from build123d import *

# Parameters (mm, degrees)
SKETCH_1_R      = 2.8
EXTRUDE_1_DEPTH = 8
SKETCH_2_W      = 18.05
SKETCH_2_H      = 18.05
EXTRUDE_2_DEPTH = 1
SKETCH_3_W      = 18.05
SKETCH_3_H      = 18.05
SKETCH_3_W_2    = 16.05
SKETCH_3_H_2    = 16.05
EXTRUDE_3_DEPTH = 9
SKETCH_6_W      = 1.2
SKETCH_6_H      = 5.825
SKETCH_6_W_2    = 5.825
SKETCH_6_H_2    = 1.2
EXTRUDE_4_DEPTH = 2.5
FILLET_3_R      = 5
FILLET_4_R      = 1.6


with BuildPart() as part:
    # 草图1 → 凸台-拉伸1 (new body)
    with BuildSketch(Plane(origin=(0, 0, 0), x_dir=(1, 0, 0), z_dir=(0, 1, 0))):
        with Locations(Location((0, 0, 0), (0, 0, 270))):
            Circle(SKETCH_1_R)
        Polygon((2.2, 0.6), (2.2, -0.6), (0.6, -0.6), (0.6, -2.2), (-0.6, -2.2), (-0.6, -0.6), (-2.2, -0.6), (-2.2, 0.6), (-0.6, 0.6), (-0.6, 2.2), (0.6, 2.2), (0.6, 0.6), align=None, mode=Mode.SUBTRACT)
    extrude(amount=-EXTRUDE_1_DEPTH)

    # 草图2 → 凸台-拉伸2 (add)
    with BuildSketch(Plane(origin=(0, 0, 0), x_dir=(1, 0, 0), z_dir=(0, 1, 0))):
        Rectangle(SKETCH_2_W, SKETCH_2_H)
    extrude(amount=EXTRUDE_2_DEPTH)

    # 草图3 → 凸台-拉伸3 (add)
    with BuildSketch(Plane(origin=(0, 0, 0), x_dir=(1, 0, 0), z_dir=(0, 1, 0))):
        Rectangle(SKETCH_3_W, SKETCH_3_H)
        Rectangle(SKETCH_3_W_2, SKETCH_3_H_2, mode=Mode.SUBTRACT)
    extrude(amount=-EXTRUDE_3_DEPTH)

    # 草图6 → 凸台-拉伸4 (add)
    with BuildSketch(Plane(origin=(0, 0, 0), x_dir=(1, 0, 0), z_dir=(0, 1, 0))):
        with Locations((0, 5.1125)):
            Rectangle(SKETCH_6_W, SKETCH_6_H)
        with Locations((5.1125, 0)):
            Rectangle(SKETCH_6_W_2, SKETCH_6_H_2)
        with Locations((0, -5.1125)):
            Rectangle(SKETCH_6_W, SKETCH_6_H)
        with Locations((-5.1125, 0)):
            Rectangle(SKETCH_6_W_2, SKETCH_6_H_2)
    extrude(amount=-EXTRUDE_4_DEPTH)

    # 圆角3
    fillet_3_edges = [part.edges().sort_by_distance(p)[0] for p in [
        (9.025, -4, 9.025),
        (9.025, -4, -9.025),
        (-9.025, -4, -9.025),
        (-9.025, -4, 9.025),
        (-8.025, -4.5, 8.025),
        (-8.025, -4.5, -8.025),
        (8.025, -4.5, -8.025),
        (8.025, -4.5, 8.025),
    ]]
    fillet(fillet_3_edges, radius=FILLET_3_R)

    # 圆角4
    fillet_4_edges = [part.edges().sort_by_distance(p)[0] for p in [
        (-8.025, 0, 1.8125),
        (-1.8125, 0, -8.025),
        (8.025, 0, -1.8125),
        (8.025, 0, 1.8125),
        (6.560533906, 0, 6.560533906),
        (-1.8125, 0, 8.025),
        (-6.560533906, 0, 6.560533906),
        (-8.025, 0, -1.8125),
        (-6.560533906, 0, -6.560533906),
        (1.8125, 0, -8.025),
        (6.560533906, 0, -6.560533906),
        (0, 1, 9.025),
        (-9.025, 1, 0),
        (9.025, 1, 0),
        (0, 1, -9.025),
        (-7.560533906, 1, -7.560533906),
        (7.560533906, 1, -7.560533906),
        (7.560533906, 1, 7.560533906),
        (-7.560533906, 1, 7.560533906),
        (1.8125, 0, 8.025),
    ]]
    fillet(fillet_4_edges, radius=FILLET_4_R)


solid = part.part
Build history of the part. All positions in model axes, mm. A direction names the side the tool comes from. Round coordinates to 2 decimals unless told otherwise and drop trailing zeros. Loops run counter-clockwise (first coordinate to the right, second up) from the corner with the lowest first, then second, coordinate; pieces in that order, holes last. Notation, with made-up numbers: (2, 46.5) -> (45, 46.5) arc R7 cw to (45, 59.5) -> close; hole circle Ø10 at (79.25, 25). An arc over 180 degrees is marked (long way). Answer in a Markdown table with one row per item.
Item 1: Drill centre lines: L1, parallel to Z at x = 3, y = -2 (3 decimals); L2, parallel to Z at x = -1.5, y = -2 (3 decimals); L3, parallel to Z at x = 1, y = -7.5 (3 decimals). Where is each one in solid material? Low to high. Write a range as [from, to].
Answers below:
| item | result |
|---|---|
| L1 | z = [-9.025, -8.025], [-0.6, 0.6], [8.025, 9.025] |
| L2 | z = [-9.025, -8.025], [-2.364, -0.6], [0.6, 2.364], [8.025, 9.025] |
| L3 | z = [-9.025, -8.025], [-2.615, -0.6], [0.6, 2.615], [8.025, 9.025] |
Item 2: Pin check, flat tips, straight feed: pin 1 (5 mm diameter, centred on x = -4.5, y = -6.5, fed in from +Z) (3 decimals); pin 2 (1.5 mm diameter, centred on y = -1.5, z = 6, fed in from +X); pin 3 (1.3 mm diameter, centred on x = 0.5, z = 0, fed in from -Y); pin 4 (2 mm diameter, centred on x = -6.5, y = -1.5, fed in from +Z). Stop position of each tip, or through.
Answers below:
| item | result |
|---|---|
| pin 1 | stops at z = 9.025 |
| pin 2 | stops at x = 8.87 |
| pin 3 | stops at y = -8 |
| pin 4 | stops at z = 8.8 |
Item 3: Saw through at B-B (z = 0). Write the cut outline in (x, y) (3 decimals), and give its area (3 significant figures).
Answers below:
| item | result |
|---|---|
| outline | (-9.025, -9) -> (-8.025, -9) -> (-8.025, -2.5) -> (-2.8, -2.5) -> (-2.8, -8) -> (-2.2, -8) -> (-2.2, 0) -> (2.2, 0) -> (2.2, -8) -> (2.8, -8) -> (2.8, -2.5) -> (8.025, -2.5) -> (8.025, -9) -> (9.025, -9) -> (9.025, -0.6) arc R1.6 ccw to (7.425, 1) -> (-7.425, 1) arc R1.6 ccw to (-9.025, -0.6) -> close |
| area | 70.7 mm² |
Item 4: Saw through at C-C (x = 0). Write the cut outline in (y, z) (3 decimals), and give its area (3 significant figures).
Answers below:
| item | result |
|---|---|
| outline | (-9, -9.025) -> (-0.6, -9.025) arc R1.6 ccw to (1, -7.425) -> (1, 7.425) arc R1.6 ccw to (-0.6, 9.025) -> (-9, 9.025) -> (-9, 8.025) -> (-2.5, 8.025) -> (-2.5, 2.8) -> (-8, 2.8) -> (-8, 2.2) -> (0, 2.2) -> (0, -2.2) -> (-8, -2.2) -> (-8, -2.8) -> (-2.5, -2.8) -> (-2.5, -8.025) -> (-9, -8.025) -> close |
| area | 70.7 mm² |
Item 5: Which spindle directions (+Z, -Z, +X, -X, +Y, -Y) get a long thin tool onto all of the face, cutting with end or side? Do faces 1 (the flat face through (5, -1, -0.6)), 2 (the cylindrical face through (-8.57, 0.52, 0.06)). Say none if no direction does.
Answers below:
| item | result |
|---|---|
| face 1 | -Y |
| face 2 | +Z, -Z, -X, +Y |
Item 6: Saw through at A-A (y = -7.5). State how many separate pieces and enclosed holes the cut face has, and give its area (3 significant figures).
Answers below:
| item | result |
|---|---|
| separate pieces | 2 |
| enclosed holes | 2 |
| area | 83.7 mm² |
Item 7: Mould opens along Z. For faces 3 (the cylindrical face through (-2.484, -3.944, 1.292)), 4 (the flat face through (-9.025, -5, 0)), 5 (the cylindrical face through (7.6, -4.86, -7.52)) say: +Z half, -Z half, draft (parallel to the pull), parting line (faces both ways), or undercut.
Answers below:
| item | result |
|---|---|
| face 3 | undercut |
| face 4 | draft |
| face 5 | -Z half |
